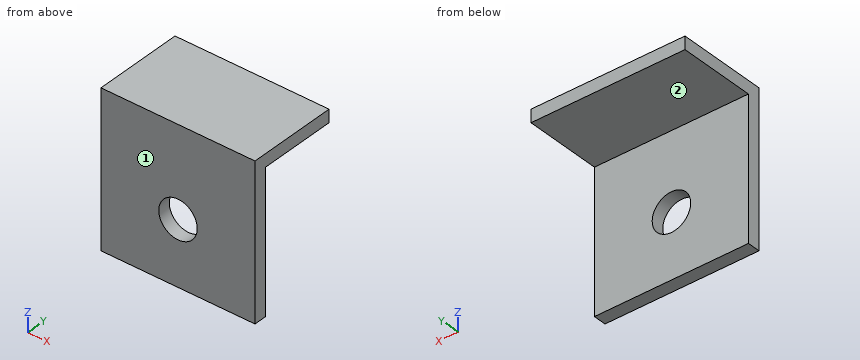
Autodesk Inventor part; units mm, degrees
ref_plane "YZ Plane" through (0, 0, 0) normal (1, 0, 0) x (0, 1, 0)
ref_plane "XZ Plane" through (0, 0, 0) normal (0, 1, 0) x (-1, 0, 0)
ref_plane "XY Plane" through (0, 0, 0) normal (0, 0, 1) x (1, 0, 0)
sketch "Sketch1" plane through (0, 0, 0) normal (1, 0, 0) x (0, 1, 0)
  line L0 (0, 0) -> (22.225, 0)
  line L1 (22.225, 0) -> (22.225, -3.175)
  line L2 (22.225, -3.175) -> (3.175, -3.175)
  line L3 (3.175, -3.175) -> (3.175, -38.1)
  line L4 (3.175, -38.1) -> (0, -38.1)
  line L5 (0, -38.1) -> (0, 0)
  dimension "d0" = 22.225
  dimension "d1" = 3.175
  dimension "d4" = 38.1
extrude "Extrusion1" add sketch "Sketch1" along normal blind 38.1
sketch "Sketch2" plane through (0, 0, -38.1) normal (0, -1, 0) x (1, 0, 0)
  circle A0 centre (19.05, 15.875) radius 4.7625
  line L0 (38.1, 38.1) -> (38.1, 0)
  point P0 (0, 38.1)
  dimension "d5" = 9.525
  dimension "d6" = 22.225
  dimension "d7" = 19.05
extrude "Extrusion2" cut sketch "Sketch2" against normal through all
properties part number "angle bracket" material "Aluminum 6061"
Work out the finished part from the listing and answer in its coordinate system (mm). Face numbers are marked on the shaded views. A direction names the side the tool comes from. Round coordinates to 2 decimals unless told otherwise and drop trailing zeros. Loops run counter-clockwise (first coordinate to the right, second up) from the corner with the lowest first, then second, coordinate; pieces in that order, holes last. Notation, with made-up numbers: M -31.75,51 L -15.75,51 A22 ccw -15.75,75 Z; hole C -3.75,42.25 d6. An arc over 180 degrees is marked long. One line per question, with ' | ' between items. Start each with the question number.
(1) Find the intervals of material crossed by line 1 (Z direction, x = 19.05, y = 0.8); line 2 (Y direction, x = 16, z = -4.5) (3 decimals); line 3 (Z direction, x = 11, y = 12.25) (3 decimals), in increasing order.
(2) A cutting plane is placed at D-D on y = 17. Write down the section's boundary in (x, z) (3 decimals).
(3) A cutting plane is placed at A-A on x = 19.05. Write down the section's boundary in (y, z) (1 decimal).
(4) A cutting plane is placed at C-C on x = 8. Write down the section's boundary in (y, z) (3 decimals), plus the area to 3 significant figures.
(5) A cutting plane is placed at B-B on z = -18. Write down the section's boundary in (x, y) (3 decimals), plus the area to 3 significant figures.
(6) Flat-ended cylindrical pins translate along their axes: pin 1 Ø12 at (x, z) = (28.5, -5) entering from +Y (3 decimals); pin 2 Ø4 at (x, z) = (18.5, -8.5) entering from +Y (3 decimals); pin 3 Ø7.5 at (x, z) = (19.05, -22.225) entering from +Y (3 decimals); pin 4 Ø9.5 at (x, y) = (22, 12) entering from -Z (3 decimals). Find the tip coordinate at first contact, or state that the pin passes through.
(7) A tool of negligible diameter and unlimited length cuts with its end or side. For the marked faces 1 and 2, from which of +Z, -Z, +X, -X, +Y, -Y can it reach the whole face along a straight path? Write none if from no direction.
Geometry check:
1) line 1: z = -38.1 to -26.99, -17.46 to 0 | line 2: y = 0 to 3.175 | line 3: z = -3.175 to 0
2) outline: M 0,-3.175 L 38.1,-3.175 L 38.1,0 L 0,0 Z
3) outline: M 0,-38.1 L 3.2,-38.1 L 3.2,-27 L 0,-27 Z; M 0,-17.5 L 3.2,-17.5 L 3.2,-3.2 L 22.2,-3.2 L 22.2,0 L 0,0 Z
4) outline: M 0,-38.1 L 3.175,-38.1 L 3.175,-3.175 L 22.225,-3.175 L 22.225,0 L 0,0 Z | area: 181 mm²
5) outline: M 0,0 L 16.852,0 L 16.852,3.175 L 0,3.175 Z; M 21.248,0 L 38.1,0 L 38.1,3.175 L 21.248,3.175 Z | area: 107 mm²
6) pin 1: stops at y = 22.225 | pin 2: stops at y = 3.175 | pin 3: passes through | pin 4: stops at z = -3.175
7) face 1: +Z, -Z, +X, -X, -Y | face 2: -Z, +X, -X, +Y
